```python
from build123d import *

# Parameters (mm, degrees)
F1_DEPTH = 304.8
F2_R     = 1.27
F4_D     = 4.318
F4_DEPTH = 25.4
F4_TIP   = 1.2972580765


with BuildPart() as f1:
    # F0 (on Top) → F1 (new body)
    with BuildSketch(Plane.XY):
        Polygon((12.7, 0), (0, 0), (-12.7, 0), (-12.7, -3.175), (-1.5875, -3.175), (-1.5875, -12.7), (0, -12.7), (1.5875, -12.7), (1.5875, -3.175), (12.7, -3.175), align=None)
    extrude(amount=F1_DEPTH)

    # F2
    f2_edges = [f1.edges().sort_by_distance(p)[0] for p in [
        (-1.5875, -3.175, 152.4),
        (1.5875, -3.175, 152.4),
    ]]
    fillet(f2_edges, radius=F2_R)

    # F4
    with Locations(Plane(origin=(0, 0, 0), x_dir=(-1, 0, 0), z_dir=(0, 1, 0))):
        with Locations((-6.35, 298.45), (-6.35, 285.75), (6.35, 285.75), (6.35, 298.45), (-6.35, 6.35), (-6.35, 19.05), (6.35, 19.05), (6.35, 6.35)):
            Hole(F4_D / 2, depth=F4_DEPTH)
            with Locations((0, 0, -(F4_DEPTH + F4_TIP / 2))):  # 118° drill point
                Cone(0, F4_D / 2, F4_TIP, mode=Mode.SUBTRACT)


solid = f1.part
```
Work out the finished part from the listing and answer in its coordinate system (mm). A direction names the side the tool comes from. Round coordinates to 2 decimals unless told otherwise and drop trailing zeros. Write each loop counter-clockwise with the first axis right and the second up, starting at its lowest first coordinate (ties: lowest second). Pieces come first, ordered by that corner, then holes.
1) A cutting plane is placed at A-A on z = 259.5. Determine the outline of the cut face in (x, y) (1 decimal), and give its area (3 significant figures).
2) Flat-ended cylindrical pins translate along their axes: P1, Ø5.5, axis at x = -6.35, z = 298.45, coming from the -Y side (3 decimals); P2, Ø6, axis at y = -7, z = 35.5, coming from the +X side; P3, Ø1, axis at y = -6.5, z = 46.5, coming from the +X side. Find the tip coordinate at first contact, or state that the pin passes through.
3) Which of the six approach directions +Z, -Z, +X, -X, +Y, -Y give full straight-line access (tool end or side, diameter ignored) to faces 1 (the face through (0, 0, 150)), 2 (the face through (-1.588, -9, 150)), 3 (the face through (1.588, -9, 150))?
4) Consider probe 1 along Z at (x, y) = (6.35, -1.65); probe 2 along X at (y, z) = (-1.8, 285.75); probe 3 along Z at (x, y) = (-5, -1.75). Determine where each line is inside the solid, lowest interval first.
Entries:
1. outline: (-12.7, -3.2) - (-2.9, -3.2) arc R1.3 cw to (-1.6, -4.4) - (-1.6, -12.7) - (1.6, -12.7) - (1.6, -4.4) arc R1.3 cw to (2.9, -3.2) - (12.7, -3.2) - (12.7, 0) - (-12.7, 0) - close
1. area: 112 mm2
2. P1: stops at y = -3.175
2. P2: stops at x = 1.67
2. P3: stops at x = 1.59
3. face 1: +Z, -Z, +X, -X, +Y
3. face 2: +Z, -Z, -X, -Y
3. face 3: +Z, -Z, +X, -Y
4. probe 1: z = 0 to 4.19, 8.51 to 16.89, 21.21 to 283.59, 287.91 to 296.29, 300.61 to 304.8
4. probe 2: x = -12.7 to -8.51, -4.19 to 4.19, 8.51 to 12.7
4. probe 3: z = 0 to 4.67, 8.03 to 17.37, 20.73 to 284.07, 287.43 to 296.77, 300.13 to 304.8
